from build123d import *

# Parameters (mm, degrees)
SKETCH1_R           = 1.7
SKETCH1_R_2         = 7
BOSS_EXTRUDE1_DEPTH = 3.175


with BuildPart() as part:
    # Sketch1 → Boss-Extrude1 (new body)
    with BuildSketch(Plane.XY):
        with BuildLine():
            Line((-1.183826785, 11.473384598), (-11.473384598, 1.183826785))
            ThreePointArc((-11.473384598, 1.183826785), (-11.616416331, 0.976858517), (-11.677035933, 0.732688077))
            ThreePointArc((-11.677035933, 0.732688077), (-11.7, 0), (-11.677035933, -0.732688077))
            ThreePointArc((-11.677035933, -0.732688077), (-11.616416331, -0.976858517), (-11.473384598, -1.183826785))
            Line((-11.473384598, -1.183826785), (-1.183826785, -11.473384598))
            ThreePointArc((-1.183826785, -11.473384598), (-0.976858517, -11.616416331), (-0.732688077, -11.677035933))
            ThreePointArc((-0.732688077, -11.677035933), (0, -11.7), (0.732688077, -11.677035933))
            ThreePointArc((0.732688077, -11.677035933), (0.976858517, -11.616416331), (1.183826785, -11.473384598))
            Line((1.183826785, -11.473384598), (11.473384598, -1.183826785))
            ThreePointArc((11.473384598, -1.183826785), (11.616416331, -0.976858517), (11.677035933, -0.732688077))
            ThreePointArc((11.677035933, -0.732688077), (11.7, 0), (11.677035933, 0.732688077))
            ThreePointArc((11.677035933, 0.732688077), (11.616416331, 0.976858517), (11.473384598, 1.183826785))
            Line((11.473384598, 1.183826785), (1.183826785, 11.473384598))
            ThreePointArc((1.183826785, 11.473384598), (0.976858517, 11.616416331), (0.732688077, 11.677035933))
            ThreePointArc((0.732688077, 11.677035933), (0, 11.7), (-0.732688077, 11.677035933))
            ThreePointArc((-0.732688077, 11.677035933), (-0.976858517, 11.616416331), (-1.183826785, 11.473384598))
        make_face()
        with Locations((0, -9)):
            Circle(SKETCH1_R, mode=Mode.SUBTRACT)
        with Locations((-9, 0)):
            Circle(SKETCH1_R, mode=Mode.SUBTRACT)
        with Locations((0, 9)):
            Circle(SKETCH1_R, mode=Mode.SUBTRACT)
        with Locations((9, 0)):
            Circle(SKETCH1_R, mode=Mode.SUBTRACT)
        Circle(SKETCH1_R_2, mode=Mode.SUBTRACT)
    extrude(amount=BOSS_EXTRUDE1_DEPTH)


solid = part.part
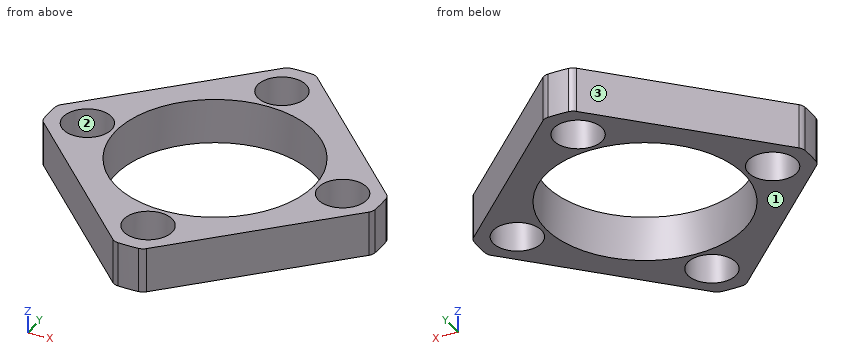
Can you work these out from the model? Positions are in its coordinate system, mm. Face numbers are marked on the shaded views. Give positions to 0.01 mm unless a question says otherwise; leave off trailing zeros. Loops run counter-clockwise (first coordinate to the right, second up) from the corner with the lowest first, then second, coordinate; pieces in that order, holes last. Notation, with made-up numbers: (19, 87) - (56, 87) arc R20 cw to (56, 115) - close; hole circle Ø9 at (-10.75, -24.75). An arc over 180 degrees is marked (long way). One line per item, written item: value.
(1) I need wall thicknesses on line 1 along Y through (x, z) = (0, 1.2); line 2 along Y through (x, z) = (1, 1.3); line 3 along X through (y, z) = (0.5, 1.9). Which ranges of each line are inside material? Lowest first, please.
Verdict:
line 1: -11.7 to -10.7, -7.3 to -7, 7 to 7.3, 10.7 to 11.7
line 2: -11.61 to -10.37, -7.63 to -6.93, 6.93 to 7.63, 10.37 to 11.61
line 3: -11.69 to -10.62, -7.38 to -6.98, 6.98 to 7.38, 10.62 to 11.69
(2) If we section it at D-D, the plane y = 9.75: List the corners of the cut face in (x, z) for me (3 decimals).
Verdict:
outline: (-2.907, 0) - (-1.526, 0) - (-1.526, 3.175) - (-2.907, 3.175) - close; (1.526, 0) - (2.907, 0) - (2.907, 3.175) - (1.526, 3.175) - close
(3) If we section it at A-A, the plane x = 0: List the corners of the cut face in (y, z) for me (3 decimals), plus the area to 4 significant figures.
Verdict:
outline: (-11.7, 0) - (-10.7, 0) - (-10.7, 3.175) - (-11.7, 3.175) - close; (-7.3, 0) - (-7, 0) - (-7, 3.175) - (-7.3, 3.175) - close; (7, 0) - (7.3, 0) - (7.3, 3.175) - (7, 3.175) - close; (10.7, 0) - (11.7, 0) - (11.7, 3.175) - (10.7, 3.175) - close
area: 8.255 mm^2
(4) I'm going to push flat-ended pins straight in: pin 1 (1 mm diameter, centred on x = 9, y = -5.5, fed in from +Z); pin 2 (1.5 mm diameter, centred on x = 5, z = 1.5, fed in from -Y); pin 3 (1.5 mm diameter, centred on y = -5.5, z = 0.5, fed in from +X). Where does each tip first touch, or does it pass through?
Verdict:
pin 1: through
pin 2: y = -8.41
pin 3: x = 7.91
(5) If we mould it in two halves opening along Y, with no side actions, what happens to the marked faces 1, 2 and 3? For each: released by +Y, released by -Y, zero draft, split by the parting line, or undercut.
Verdict:
face 1: zero draft
face 2: undercut
face 3: released by +Y
(6) If we section it at C-C, the plane z = 2.05: List the corners of the cut face in (x, y) for me, plus the area to 3 significant figures.
Verdict:
outline: (-11.68, -0.73) arc R0.7 ccw to (-11.47, -1.18) - (-1.18, -11.47) arc R0.7 ccw to (-0.73, -11.68) arc R11.7 ccw to (0.73, -11.68) arc R0.7 ccw to (1.18, -11.47) - (11.47, -1.18) arc R0.7 ccw to (11.68, -0.73) arc R11.7 ccw to (11.68, 0.73) arc R0.7 ccw to (11.47, 1.18) - (1.18, 11.47) arc R0.7 ccw to (0.73, 11.68) arc R11.7 ccw to (-0.73, 11.68) arc R0.7 ccw to (-1.18, 11.47) - (-11.47, 1.18) arc R0.7 ccw to (-11.68, 0.73) arc R11.7 ccw to start; hole circle Ø3.4 at (-9, 0); hole circle Ø14 at (0, 0); hole circle Ø3.4 at (0, -9); hole circle Ø3.4 at (0, 9); hole circle Ø3.4 at (9, 0)
area: 126 mm^2
